```python
from build123d import *

# Parameters (mm, degrees)
SKETCH_1_W      = 80
SKETCH_1_H      = 28
SKETCH_1_R      = 4.25
SKETCH_1_R_2    = 2
EXTRUDE_1_DEPTH = 3
FILLET_1_RADIUS = 14
FILLET_1_LENGTH = 3
FILLET_2_RADIUS = 14
FILLET_2_LENGTH = 3


with BuildPart() as part:
    # 草图1 → 凸台-拉伸1 (new body)
    with BuildSketch(Plane(origin=(0, 0, 0), x_dir=(1, 0, 0), z_dir=(0, 1, 0))):
        Rectangle(SKETCH_1_W, SKETCH_1_H)
        with Locations(Location((25, 0, 0), (0, 0, 270))):
            Circle(SKETCH_1_R, mode=Mode.SUBTRACT)
        with Locations(Location((-25, 0, 0), (0, 0, 270))):
            Circle(SKETCH_1_R_2, mode=Mode.SUBTRACT)
    extrude(amount=EXTRUDE_1_DEPTH)

    # 圆角1: full round fillet: the end face becomes a half cylinder, R = half its width
    fillet_1_face = Plane((-40, 1.5, 0), x_dir=(0, 1, 0), z_dir=(-1, 0, 0))  # on the end face: x along it, z out of the body
    fillet_1_slab = fillet_1_face.offset(-FILLET_1_RADIUS / 2) * Box(FILLET_1_LENGTH, 2 * FILLET_1_RADIUS, FILLET_1_RADIUS, mode=Mode.PRIVATE)  # the body's end, R deep
    fillet_1_round = Plane((-26, 1.5, 0), x_dir=(-1, 0, 0), z_dir=(0, 1, 0)) * Cylinder(FILLET_1_RADIUS, FILLET_1_LENGTH, mode=Mode.PRIVATE)  # its axis R under the face
    add(fillet_1_slab - fillet_1_round, mode=Mode.SUBTRACT)

    # 圆角2: full round fillet: the end face becomes a half cylinder, R = half its width
    fillet_2_face = Plane((40, 1.5, 0), x_dir=(0, -1, 0), z_dir=(1, 0, 0))  # on the end face: x along it, z out of the body
    fillet_2_slab = fillet_2_face.offset(-FILLET_2_RADIUS / 2) * Box(FILLET_2_LENGTH, 2 * FILLET_2_RADIUS, FILLET_2_RADIUS, mode=Mode.PRIVATE)  # the body's end, R deep
    fillet_2_round = Plane((26, 1.5, 0), x_dir=(1, 0, 0), z_dir=(0, -1, 0)) * Cylinder(FILLET_2_RADIUS, FILLET_2_LENGTH, mode=Mode.PRIVATE)  # its axis R under the face
    add(fillet_2_slab - fillet_2_round, mode=Mode.SUBTRACT)


solid = part.part
```
Here's how the part is built. I have some questions about the finished solid (model axes, mm). Give positions to 0.01 mm unless a question says otherwise; leave off trailing zeros. Loops run counter-clockwise (first coordinate to the right, second up) from the corner with the lowest first, then second, coordinate; pieces in that order, holes last. Notation, with made-up numbers: M 70.5,70.25 L 104.5,70.25 A23 ccw 104.5,81.25 Z; hole C 70,-3.75 d10. An arc over 180 degrees is marked long. Put each result on its own line as item: value. Start each with the question number.
(1) If we mould it in two halves opening along Z, with no side actions, what happens to faces 1 (the cylindrical face through (40, 1, 0)), 2 (the flat face through (0, 1, 14)), 3 (the cylindrical face through (29.214, 1.479, -0.553))? For each: +Z half, -Z half, draft (parallel to the pull), parting line (faces both ways), or undercut.
(2) I want a section at B-B on x = 25. Please give me the cut outline in (y, z).
(3) I want a section at C-C on y = 1.2. Please give me the cut outline in (x, z).
(4) I want a section at A-A on z = 0. Please give me the cut outline in (x, y).
(5) I want a section at D-D on z = 5.5. Please give me the cut outline in (x, y).
(6) I need wall thicknesses on line 1 along X through (y, z) = (1.55, 0); line 2 along X through (y, z) = (2.4, -1.5); line 3 along Z through (x, y) = (31.5, 1.9). Which ranges of each line are inside material? Lowest first, please. Write a range as [from, to].
Answer block:
1. face 1: parting line
1. face 2: +Z half
1. face 3: undercut
2. outline: M 0,-14 L 3,-14 L 3,-4.25 L 0,-4.25 Z; M 0,4.25 L 3,4.25 L 3,14 L 0,14 Z
3. outline: M -26,-14 L 26,-14 A14 ccw 26,14 L -26,14 A14 ccw Z; hole C -25,0 d4; hole C 25,0 d8.5
4. outline: M -40,0 L -27,0 L -27,3 L -40,3 Z; M -23,0 L 20.75,0 L 20.75,3 L -23,3 Z; M 29.25,0 L 40,0 L 40,3 L 29.25,3 Z
5. outline: M -38.87,0 L 38.87,0 L 38.87,3 L -38.87,3 Z
6. line 1: [-40, -27], [-23, 20.75], [29.25, 40]
6. line 2: [-39.92, -26.32], [-23.68, 21.02], [28.98, 39.92]
6. line 3: [-12.87, 12.87]
